Part model, mm, in its own coordinate system. A direction names the side the tool comes from. Coordinates: 2 decimals unless noted, no trailing zeros. Loops run counter-clockwise (first coordinate to the right, second up) from the corner with the lowest first, then second, coordinate; pieces in that order, holes last. Notation, with made-up numbers: M 28,16.5 L 61,16.5 A18 cw 61,47.5 Z; hole C 64,68 d7. An arc over 180 degrees is marked long. Answer as a JSON object with one key per item and string values. Group by question number.
1. Saw through at A-A on z = 4. Write the cut outline in (x, y), then the cut area to 3 significant figures.
2. Saw through at B-B on y = 11. Write the cut outline in (x, z).
3. Drill centre lines: L1, parallel to Y at x = 24.5, z = 4.75; L2, parallel to Z at x = 19.5, y = 4. Where is each one in solid material? Low to high.
4. Saw through at D-D on y = 2.5. Write the cut outline in (x, z).
5. Drop a flat-ended pin along its axis: pin 1 Ø2.5 at (x, y) = (4, 19.91) entering from +Z. Give the stop position or say it passes through.
6. Saw through at C-C on x = 19. Write the cut outline in (y, z).
7. Mould opens along Y. For faces 4 (the face through (8.1, 15, 1)), 5 (the face through (2.31, 38.52, 5.67)) say: released by +Y, released by -Y, zero draft, split by the parting line, or undercut.
8. 3-axis set-ups, long thin cutter, end or side, ignore diameter. For faces 1 (the face through (19, 16, 0)), 2 (the face through (8.722, 24.207, 0.986)), 3 (the face through (13, 3, 6)): which of +Z, -Z, +X, -X, +Y, -Y reach the whole face in a straight line?
Autodesk Fusion 360 part; units mm, degrees
sketch "Sketch1" plane through (0, 0, 0) normal (0, 0, 1) x (1, 0, 0)
  line L0 (0, 0) -> (26, 0)
  line L1 (26, 0) -> (26, 40)
  line L2 (26, 40) -> (0, 40)
  line L3 (0, 40) -> (0, 0)
  dimension "d1" = 26
  dimension "d2" = 40
sketch "Sketch2" plane through (0, 0, 0) normal (0, 0, 1) x (1, 0, 0)
  circle A0 centre (23, 10) radius 1.5
  circle A1 centre (3, 10) radius 1.5
  line L0 (26, 0) -> (26, 40)
  circle A2 centre (23, 30) radius 1.5
  circle A3 centre (3.0002, 29.9091) radius 1.5
  line L1 (26, 40) -> (0, 40)
  circle A4 centre (13.0002, 28.9091) radius 1
  circle A5 centre (4.0002, 19.9091) radius 1
  circle A6 centre (13, 11) radius 1
  circle A7 centre (22, 20) radius 1
  line L2 (6.2078, 21.6931) -> (11.3069, 26.7922)
  arc A8 (6.2078, 21.6931) -> (14.6931, 13.2078) centre (13, 20) ccw
  arc A9 (19.7922, 18.3069) -> (11.3069, 26.7922) centre (13, 20) ccw
  line L3 (19.7922, 18.3069) -> (14.6931, 13.2078)
  dimension "d3" = 3
  dimension "d4" = 3
  dimension "d5" = 3
  dimension "d6" = 20
  dimension "d7" = 3
  dimension "d8" = 3
  dimension "d9" = 20
  dimension "d10" = 3
  dimension "d11" = 20
  dimension "d12" = 10
  dimension "d14" = 10
  dimension "d15" = 1
  dimension "d16" = 2
  dimension "d17" = 2
  dimension "d18" = 2
  dimension "d19" = 10
  dimension "d20" = 1
  dimension "d21" = 10
  dimension "d22" = 1
  dimension "d24" = 10
  dimension "d25" = 1
extrude "Extrude1" add sketch "Sketch1" along normal blind 2
extrude "Extrude2" cut sketch "Sketch2" along normal blind 2
sketch "Sketch3" plane through (0, 0, 2) normal (0, 0, 1) x (-1, 0, 0)
  circle A0 centre (-13.0002, -28.9091) radius 1
  circle A1 centre (-23, -10) radius 1.5
  circle A2 centre (-3, -10) radius 1.5
  circle A3 centre (-3.0002, -29.9091) radius 1.5
  circle A4 centre (-23, -30) radius 1.5
  line L0 (-6.2078, -21.6931) -> (-11.3069, -26.7922)
  arc A5 (-19.7922, -18.3069) -> (-11.3069, -26.7922) centre (-13, -20) ccw
  line L1 (-19.7922, -18.3069) -> (-14.6931, -13.2078)
  arc A6 (-6.2078, -21.6931) -> (-14.6931, -13.2078) centre (-13, -20) ccw
  circle A7 centre (-13, -11) radius 1
  circle A8 centre (-4.0002, -19.9091) radius 1
  circle A9 centre (-22, -20) radius 1
  line L2 (0, -40) -> (0, 0)
  line L3 (0, 0) -> (-26, 0)
  line L4 (-26, 0) -> (-26, -40)
  line L5 (-26, -40) -> (0, -40)
  line L6 (0, 0) -> (-26, 0)
  line L7 (-26, 0) -> (-26, -3)
  line L8 (-26, -3) -> (0, -3)
  line L9 (0, -3) -> (0, 0)
  line L10 (0, -40) -> (-26, -40)
  line L11 (-26, -40) -> (-26, -37)
  line L12 (-26, -37) -> (0, -37)
  line L13 (0, -37) -> (0, -40)
extrude "Extrude3" add sketch "Sketch3" along normal blind 8 contours L2 L4 L5 L10 L11 L12 L13 | L2 L3 L4 L6 L7 L8 L9
sketch "Sketch4" plane through (0, 0, 0) normal (0, -1, 0) x (1, 0, 0)
  line L0 (0, 0) -> (26, 0)
  line L1 (26, 0) -> (26, 10)
  line L2 (26, 10) -> (0, 10)
  line L3 (0, 10) -> (0, 0)
  circle A0 centre (23, 7) radius 1.5
  circle A1 centre (3, 7) radius 1.5
  dimension "d41" = 3
  dimension "d42" = 3
  dimension "d43" = 3
  dimension "d44" = 3
  dimension "d45" = 20
extrude "Extrude4" cut sketch "Sketch4" against normal blind 3 contours A0 | A1
sketch "Sketch5" plane through (0, 40, 0) normal (0, 1, 0) x (-1, 0, 0)
  line L0 (-26, 0) -> (0, 0)
  line L1 (0, 0) -> (0, 10)
  line L2 (0, 10) -> (-26, 10)
  line L3 (-26, 10) -> (-26, 0)
  circle A0 centre (-3, 7) radius 1.5
  circle A1 centre (-23, 7) radius 1.5
  dimension "d48" = 3
  dimension "d49" = 3
  dimension "d50" = 20
  dimension "d51" = 3
  dimension "d52" = 3
  dimension "d53" = 3
extrude "Extrude5" cut sketch "Sketch5" against normal blind 3 contours A0 | A1
Outcome:
{
 "1": {"outline": "M 0,0 L 26,0 L 26,3 L 0,3 Z; M 0,37 L 26,37 L 26,40 L 0,40 Z", "area": "156 mm²"},
 "2": {"outline": "M 0,0 L 1.88,0 L 1.88,2 L 0,2 Z; M 4.12,0 L 12,0 L 12,2 L 4.12,2 Z; M 14,0 L 21.88,0 L 21.88,2 L 14,2 Z; M 24.12,0 L 26,0 L 26,2 L 24.12,2 Z"},
 "3": {"L1": "y = 0 to 3, 37 to 40", "L2": "z = 0 to 2"},
 "4": {"outline": "M 0,0 L 26,0 L 26,10 L 0,10 Z; hole C 3,7 d3; hole C 23,7 d3"},
 "5": {"pin 1": "stops at z = 2"},
 "6": {"outline": "M 0,0 L 17.51,0 L 17.51,2 L 3,2 L 3,10 L 0,10 Z; M 23.61,0 L 40,0 L 40,10 L 37,10 L 37,2 L 23.61,2 Z"},
 "7": {"face 4": "undercut", "face 5": "zero draft"},
 "8": {"face 1": "-Z, +X, -X, +Y, -Y", "face 2": "+Z, -Z", "face 3": "+Z, +X, -X"}
}
